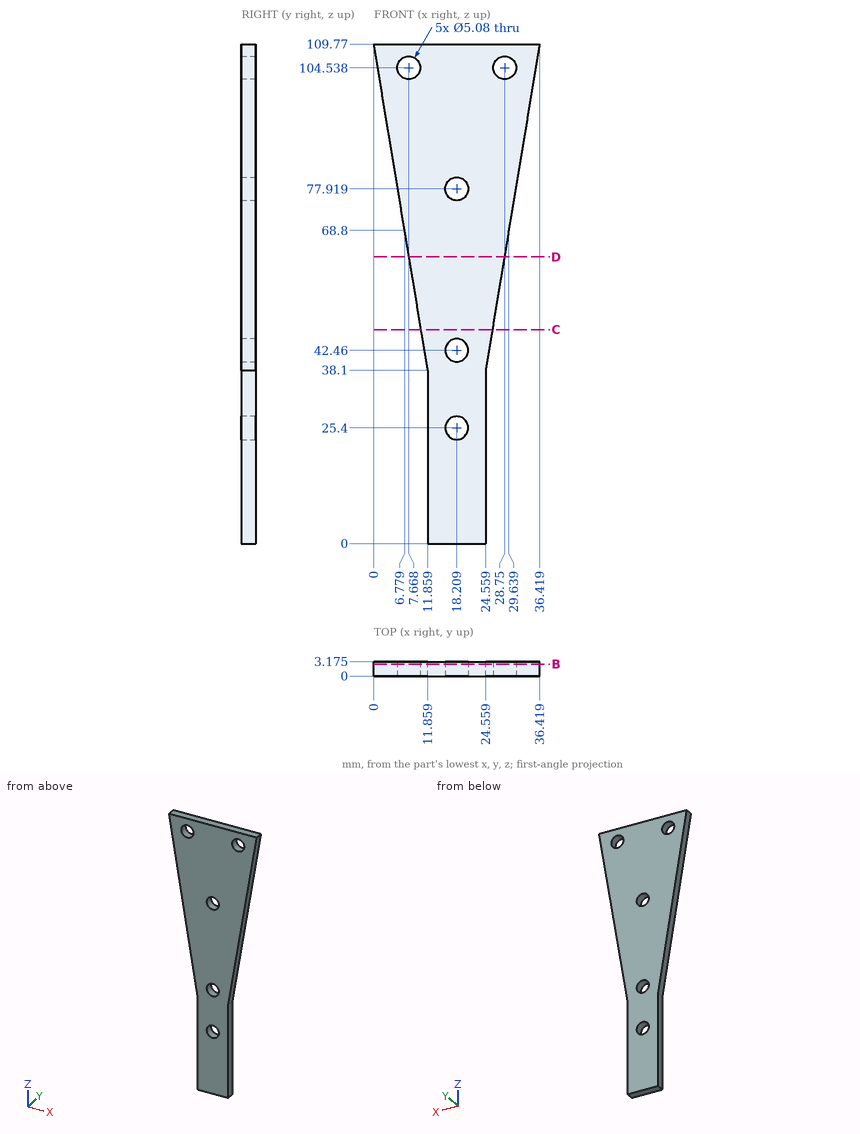
Design review of the part shown in the three views and the two pictorial views. Dimensions are in mm from the part's minimum x, y and z. Round coordinates to 2 decimals unless told otherwise and drop trailing zeros. Loops run counter-clockwise (first coordinate to the right, second up) from the corner with the lowest first, then second, coordinate; pieces in that order, holes last. Notation, with made-up numbers: (47, -25.5) -> (54, -25.5) arc R9 cw to (54, -20.5) -> close; hole circle Ø6 at (36.25, 7). An arc over 180 degrees is marked (long way). Use one line per item in the form item = value. Start each with the question number.
Q1. We need section B-B on y = 2.6. Give the boundary of the cut face in (x, z).
Q2. For pin 1 Ø3 at (x, z) = (18.21, 25.4) entering from +Y; pin 2 Ø1.5 at (y, z) = (2.5, 93.5) entering from +X; pin 3 Ø1.6 at (y, z) = (1, 17.5) entering from +X; pin 4 Ø1 at (y, z) = (2, 14.5) entering from -X, all flat-tipped, find the tip position at first contact; note any pin that passes through.
Q3. We need section C-C on z = 47. Give the boundary of the cut face in (x, y) (1 decimal).
Q4. We need section D-D on z = 63. Give the boundary of the cut face in (x, y) (1 decimal).
Q5. Wall thickness on line 1 along X through (y, z) = (0.4, 13); line 2 along Z through (x, y) = (19, 1.9) (1 decimal); line 3 along X through (y, z) = (1.1, 27) (1 decimal): over which ranges is each line inside the solid? List them lowest first. Write a range as [from, to].
Calculated:
q1.outline = (0, 109.77) -> (11.86, 38.1) -> (11.86, 0) -> (24.56, 0) -> (24.56, 38.1) -> (36.42, 109.77) -> close; hole circle Ø5.08 at (7.67, 104.54); hole circle Ø5.08 at (18.21, 25.4); hole circle Ø5.08 at (18.21, 42.46); hole circle Ø5.08 at (18.21, 77.92); hole circle Ø5.08 at (28.75, 104.54)
q2.pin_1 = through
q2.pin_2 = 33.85
q2.pin_3 = 24.56
q2.pin_4 = 11.86
q3.outline = (10.4, 0) -> (26, 0) -> (26, 3.2) -> (10.4, 3.2) -> close
q4.outline = (7.7, 0) -> (28.7, 0) -> (28.7, 3.2) -> (7.7, 3.2) -> close
q5.line_1 = [11.86, 24.56]
q5.line_2 = [0, 23], [27.8, 40], [44.9, 75.5], [80.3, 109.8]
q5.line_3 = [11.9, 16.2], [20.2, 24.6]
